```python
from build123d import *

# Parameters (mm, degrees)
SKETCH1_R           = 3.8
BOSS_EXTRUDE1_DEPTH = 5
FILLET1_R           = 10


with BuildPart() as part:
    # Sketch1 → Boss-Extrude1 (new body)
    with BuildSketch(Plane.XY):
        Polygon((-12.5, 15), (-12.5, -15), (-10, -15), (-10, -20), (-5, -20), (-5, -15), (-1.5, -15), (-1.5, -12), (-2.6, -12), (-2.6, -9.7), (-1.5, -9.7), (-1.5, -5), (1.5, -5), (1.5, -9.7), (2.6, -9.7), (2.6, -12), (1.5, -12), (1.5, -15), (5, -15), (5, -20), (10, -20), (10, -15), (12.5, -15), (12.5, 15), align=None)
        with Locations((0, 5)):
            Circle(SKETCH1_R, mode=Mode.SUBTRACT)
    extrude(amount=BOSS_EXTRUDE1_DEPTH)

    # Fillet1
    fillet1_edges = [part.edges().sort_by_distance(p)[0] for p in [
        (-12.5, 15, 2.5),
        (12.5, 15, 2.5),
    ]]
    fillet(fillet1_edges, radius=FILLET1_R)


solid = part.part
```
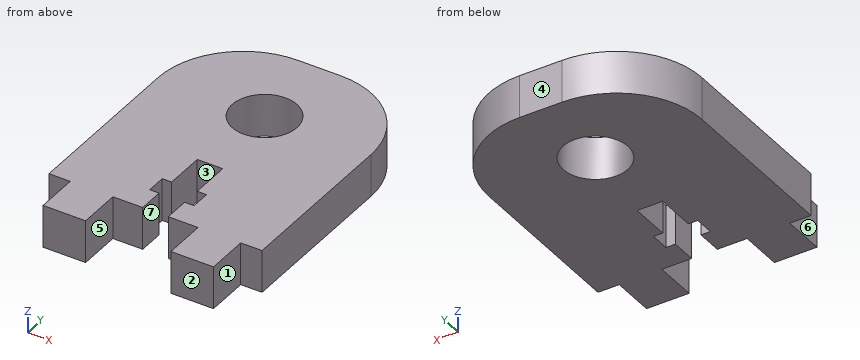
Check sheet for the modelled part. Datum: model origin and axes. Units: mm. Face numbers are marked on the shaded views. A direction names the side the tool comes from. Round coordinates to 2 decimals unless told otherwise and drop trailing zeros. Write each loop counter-clockwise with the first axis right and the second up, starting at its lowest first coordinate (ties: lowest second). Pieces come first, ordered by that corner, then holes. Notation, with made-up numbers: (-3.75, -25.5) -> (41.25, -25.5) arc R29 cw to (41.25, -3.5) -> close; hole circle Ø3 at (55.5, 30). An arc over 180 degrees is marked (long way). One line per question, with ' | ' between items. Start each with the question number.
1. Sectioned sample at D-D, the plane x = -10.5. Record the cut outline in (y, z).
2. Sectioned sample at A-A, the plane y = -7.5. Record the cut outline in (x, z).
3. Sectioned sample at C-C, the plane z = 3. Record the cut outline in (x, y), then the cut area to 3 significant figures.
4. Depth check by flat-ended pin: pin 1 (3 mm diameter, centred on x = 4, z = 1.5, fed in from -Y); pin 2 (2 mm diameter, centred on x = -11.5, z = 2.5, fed in from -Y); pin 3 (2.5 mm diameter, centred on y = -18, z = 3.5, fed in from +X); pin 4 (0.9 mm diameter, centred on x = 0.5, z = 2, fed in from -Y). Enter the tip coordinate at first touch or a pass-through.
5. Release check for a two-part mould opening along X. For the marked faces 4, 5, 6 and 7 record: +X half, -X half, draft (parallel to the pull), parting line (faces both ways), or undercut.
6. Set-up check for the marked faces 1, 2 and 3: record each of +Z, -Z, +X, -X, +Y, -Y from which the full face is reachable in a straight line by a thin tool's end or side.
7. Scan lines: line 1 along Y through (x, z) = (0, 3.8); line 2 along Y through (x, z) = (-2, 4.45); line 3 along X through (y, z) = (-9.5, 2.9). Record each from-to range of solid material in increasing order. Write a range as from..to.
8. Sectioned sample at B-B, the plane x = 0. Record the cut outline in (y, z).
Taken from the geometry:
1) outline: (-15, 0) -> (11, 0) -> (11, 5) -> (-15, 5) -> close
2) outline: (-12.5, 0) -> (-1.5, 0) -> (-1.5, 5) -> (-12.5, 5) -> close; (1.5, 0) -> (12.5, 0) -> (12.5, 5) -> (1.5, 5) -> close
3) outline: (-12.5, -15) -> (-10, -15) -> (-10, -20) -> (-5, -20) -> (-5, -15) -> (-1.5, -15) -> (-1.5, -12) -> (-2.6, -12) -> (-2.6, -9.7) -> (-1.5, -9.7) -> (-1.5, -5) -> (1.5, -5) -> (1.5, -9.7) -> (2.6, -9.7) -> (2.6, -12) -> (1.5, -12) -> (1.5, -15) -> (5, -15) -> (5, -20) -> (10, -20) -> (10, -15) -> (12.5, -15) -> (12.5, 5) arc R10 ccw to (2.5, 15) -> (-2.5, 15) arc R10 ccw to (-12.5, 5) -> close; hole circle Ø7.6 at (0, 5) | area: 677 mm^2
4) pin 1: stops at y = -20 | pin 2: stops at y = -15 | pin 3: stops at x = 10 | pin 4: stops at y = -5
5) face 4: draft | face 5: undercut | face 6: -X half | face 7: undercut
6) face 1: +Z, -Z, +X, -Y | face 2: +Z, -Z, +X, -X, -Y | face 3: +Z, -Z, -Y
7) line 1: y = -5..1.2, 8.8..15 | line 2: y = -15..-12, -9.7..1.77, 8.23..15 | line 3: x = -12.5..-1.5, 1.5..12.5
8) outline: (-5, 0) -> (1.2, 0) -> (1.2, 5) -> (-5, 5) -> close; (8.8, 0) -> (15, 0) -> (15, 5) -> (8.8, 5) -> close
